Part model, mm, in its own coordinate system. Coordinates: 2 decimals unless noted, no trailing zeros. Loops run counter-clockwise (first coordinate to the right, second up) from the corner with the lowest first, then second, coordinate; pieces in that order, holes last. Notation, with made-up numbers: (80, 65.5) -> (131, 65.5) arc R14 ccw to (131, 91.5) -> close; hole circle Ø2 at (77, 4.25). An arc over 180 degrees is marked (long way). One line per question, with ' | ' between items. Start each with the question number.
1) Cut at B-B (y = 0). List the corners of the cut face in (x, z).
2) Probe L1, parallel to Y at x = -40, z = 1.05; L2, parallel to Y at x = 0, z = -0.85; L3, parallel to X at y = 2, z = 1.55. List the from-to ranges inside material, lowest first. Write a range as from..to.
3) Cut at C-C (x = 40). List the corners of the cut face in (y, z), plus the area to 4 significant figures.
4) Drop a flat-ended pin along its axis: pin 1 (7 mm diameter, centred on x = 0, y = 80, fed in from -Z). Give the stop position or say it passes through.
5) Cut at D-D (y = 80). List the corners of the cut face in (x, z).
6) Cut at A-A (z = 0). List the corners of the cut face in (x, y).
Autodesk Inventor part; units mm, degrees
ref_plane "YZ Plane" through (0, 0, 0) normal (1, 0, 0) x (0, 1, 0)
ref_plane "XZ Plane" through (0, 0, 0) normal (0, 1, 0) x (-1, 0, 0)
ref_plane "XY Plane" through (0, 0, 0) normal (0, 0, 1) x (1, 0, 0)
sketch "Sketch1" plane through (0, 0, 0) normal (0, 0, 1) x (1, 0, 0)
  circle A0 centre (0, 0) radius 4.25
  circle A1 centre (-40, 0) radius 4.25
  circle A2 centre (40, 0) radius 4.25
  circle A3 centre (0, 80) radius 4.25
  circle A4 centre (0, 40) radius 4.25
  line L0 (0, 0) -> (0, 80) construction
  line L1 (-40, 0) -> (40, 0) construction
  line L2 (-58, 98) -> (58, 98)
  line L3 (58, 98) -> (58, -18)
  line L4 (58, -18) -> (-58, -18)
  line L5 (-58, -18) -> (-58, 98)
  line L6 (-58, 98) -> (58, -18) construction
  line L7 (58, 98) -> (-58, -18) construction
  line L8 (-58, 22) -> (-20, 98)
  line L9 (20, 98) -> (58, 22)
  dimension "d0" = 8.5
  dimension "d1" = 8.5
  dimension "d2" = 8.5
  dimension "d3" = 8.5
  dimension "d4" = 8.5
  dimension "d5" = 80
  dimension "d6" = 80
  dimension "d7" = 116
  dimension "d8" = 116
  dimension "d9" = 40
  dimension "d10" = 40
  dimension "d11" = 40
extrude "Extrusion1" add sketch "Sketch1" along normal mid plane 5 contours L2 L9 L3 L4 L5 L8
fillet "Fillet1" radius 3 6 edges at (-58, -18, 0) (-58, 22, 0) (20, 98, 0) (-20, 98, 0) (58, 22, 0) (58, -18, 0)
equation "\"d1\" = d0"
equation "\"d2\" = d0"
equation "\"d3\" = d0"
equation "\"d4\" = d0"
properties part number "Connection_plate_T_120x120" material "Aluminum 6061"
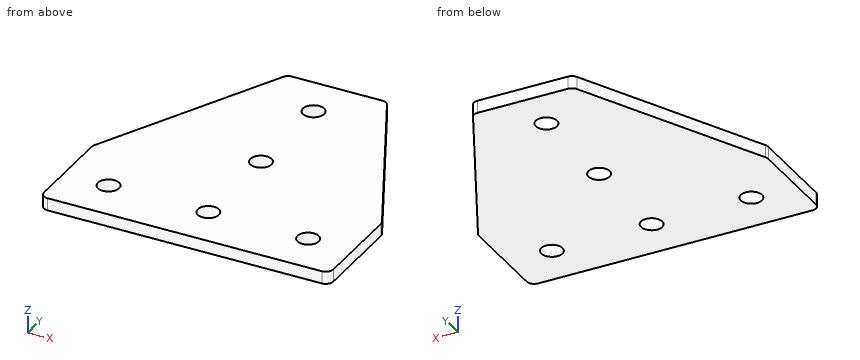
Reported:
1) outline: (-58, -2.5) -> (-44.25, -2.5) -> (-44.25, 2.5) -> (-58, 2.5) -> close; (-35.75, -2.5) -> (-4.25, -2.5) -> (-4.25, 2.5) -> (-35.75, 2.5) -> close; (4.25, -2.5) -> (35.75, -2.5) -> (35.75, 2.5) -> (4.25, 2.5) -> close; (44.25, -2.5) -> (58, -2.5) -> (58, 2.5) -> (44.25, 2.5) -> close
2) L1: y = -18..-4.25, 4.25..58 | L2: y = -18..-4.25, 4.25..35.75, 44.25..75.75, 84.25..98 | L3: x = -58..-43.75, -36.25..-3.75, 3.75..36.25, 43.75..58
3) outline: (-18, -2.5) -> (-4.25, -2.5) -> (-4.25, 2.5) -> (-18, 2.5) -> close; (4.25, -2.5) -> (58, -2.5) -> (58, 2.5) -> (4.25, 2.5) -> close | area: 337.5 mm²
4) pin 1: passes through
5) outline: (-29, -2.5) -> (-4.25, -2.5) -> (-4.25, 2.5) -> (-29, 2.5) -> close; (4.25, -2.5) -> (29, -2.5) -> (29, 2.5) -> (4.25, 2.5) -> close
6) outline: (-58, -15) arc R3 ccw to (-55, -18) -> (55, -18) arc R3 ccw to (58, -15) -> (58, 21.29) arc R3 ccw to (57.68, 22.63) -> (20.83, 96.34) arc R3 ccw to (18.15, 98) -> (-18.15, 98) arc R3 ccw to (-20.83, 96.34) -> (-57.68, 22.63) arc R3 ccw to (-58, 21.29) -> close; hole circle Ø8.5 at (-40, 0); hole circle Ø8.5 at (0, 0); hole circle Ø8.5 at (0, 40); hole circle Ø8.5 at (0, 80); hole circle Ø8.5 at (40, 0)
